Design review of the part built by this model. Coordinates are the model's own, in mm. A direction names the side the tool comes from. Coordinates: 2 decimals unless noted, no trailing zeros. Order: outer loops, then holes, each group sorted by start corner. A loop starts at its lowest first (then second) coordinate and runs counter-clockwise, first axis right, second up. Notation, with made-up numbers: M -27.75,-20.5 L 9.25,-20.5 A14 cw 9.25,-8.5 Z; hole C -28,20.5 d4. An arc over 180 degrees is marked long. Use CSV: the item, a comma, the result in double quotes.
```python
from build123d import *

# Parameters (mm, degrees)
SKETCH1_W           = 6.8
SKETCH1_H           = 12
SKETCH1_W_2         = 2.8
SKETCH1_H_2         = 8
BOSS_EXTRUDE2_DEPTH = 2.7
SKETCH2_W           = 6.8
SKETCH2_H           = 12
BOSS_EXTRUDE3_DEPTH = 0.4
SKETCH3_W           = 3
SKETCH3_H           = 9
CUT_EXTRUDE1_DEPTH  = 26.413775792


with BuildPart() as part:
    # Sketch1 → Boss-Extrude2 (new body)
    with BuildSketch(Plane.XY):
        with Locations((-21.1, 0)):
            Rectangle(SKETCH1_W, SKETCH1_H)
        with Locations((-21.1, 0)):
            Rectangle(SKETCH1_W_2, SKETCH1_H_2, mode=Mode.SUBTRACT)
    extrude(amount=BOSS_EXTRUDE2_DEPTH)

    # Sketch2 → Boss-Extrude3 (add)
    with BuildSketch(Plane.XY.offset(2.7)):
        with Locations((-21.1, 0)):
            Rectangle(SKETCH2_W, SKETCH2_H)
    extrude(amount=BOSS_EXTRUDE3_DEPTH)

    # Sketch3 → Cut-Extrude1 (cut, through all)
    with BuildSketch(Plane.XY.offset(3.1)):
        with Locations((-19.2, 0)):
            Rectangle(SKETCH3_W, SKETCH3_H)
    extrude(amount=-CUT_EXTRUDE1_DEPTH, mode=Mode.SUBTRACT)


solid = part.part
```
(1) Add section C-C on x = -21.25. State the section outline as (y, z) points.
The answers:
outline,"M -6,0 L -4,0 L -4,2.7 L 4,2.7 L 4,0 L 6,0 L 6,3.1 L -6,3.1 Z"
(2) Wall thickness on probe 1 along Y at (x, z) = (-18.75, 2.1); probe 2 along Y at (x, z) = (-21, 1.1); probe 3 along Z at (x, y) = (-21.5, -0.5): over which ranges is each line inside the solid? List them lowest first.
The answers:
probe 1,"y = -6 to -4.5, 4.5 to 6"
probe 2,"y = -6 to -4, 4 to 6"
probe 3,"z = 2.7 to 3.1"
(3) The part is to be moulded in two halves that separate along Y. For faces 4 (the face through (-22.5, 0, 1)), 5 (the face through (-17.7, -5, 2)), 6 (the face through (-21, 6, 2)), say which applies: pulls with the +Y half, pulls with the -Y half, needs draft (parallel to the pull), parting line crosses it, or undercut.
The answers:
face 4,"undercut"
face 5,"needs draft"
face 6,"pulls with the +Y half"
(4) Add section A-A on x = -18.5. State the section outline as (y, z) points.
The answers:
outline,"M -6,0 L -4.5,0 L -4.5,3.1 L -6,3.1 Z; M 4.5,0 L 6,0 L 6,3.1 L 4.5,3.1 Z"
(5) Add section B-B on z = 2.9. State the section outline as (x, y) points.
The answers:
outline,"M -24.5,-6 L -17.7,-6 L -17.7,-4.5 L -20.7,-4.5 L -20.7,4.5 L -17.7,4.5 L -17.7,6 L -24.5,6 Z"
(6) For faces 1 (the face through (-22, 0, 3.1)), 2 (the face through (-22, 4, 1)), 3 (the face through (-19, -4.5, 2)), list the 3-axis set-ups (+Z, -Z, +X, -X, +Y, -Y) from which the entire face can be reached by the end or side of a thin tool; tool diameter is ignored.
The answers:
face 1,"+Z, +X, -X, +Y, -Y"
face 2,"-Z, +X"
face 3,"+Z, -Z, +X"
(7) Clearance check with flat-ended pins moving along their axes: P1, Ø2, axis at x = -18.5, y = 3, coming from the +Z side; P2, Ø1, axis at x = -20.5, y = -3, coming from the -Z side; P3, Ø1.5, axis at y = 1, z = 0.5, coming from the +X side. State where each tip first meets the part, or that it passes through.
The answers:
P1,"passes through"
P2,"stops at z = 2.7"
P3,"stops at x = -22.5"
(8) Add section D-D on y = -0.75. State the section outline as (x, z) points, and give its area (3 significant figures).
The answers:
outline,"M -24.5,0 L -22.5,0 L -22.5,2.7 L -20.7,2.7 L -20.7,3.1 L -24.5,3.1 Z"
area,"6.92 mm2"
